Part model, mm, in its own coordinate system. Coordinates: 2 decimals unless noted, no trailing zeros. Loops run counter-clockwise (first coordinate to the right, second up) from the corner with the lowest first, then second, coordinate; pieces in that order, holes last. Notation, with made-up numbers: (-14, 51.25) -> (-4, 51.25) arc R22 cw to (-4, 65.25) -> close; hole circle Ø10 at (0.5, -38.5). An arc over 180 degrees is marked (long way). Use one line per item in the form item = value. Start each with the question number.
(1) Band-saw the part on D-D on z = 15.24. Give the cut face in (x, y) (3 decimals).
(2) Band-saw the part on C-C on x = 0. Give the cut face in (y, z) (3 decimals).
(3) Band-saw the part on A-A on z = 189. Give the cut face in (x, y) (3 decimals), then the cut area to 3 significant figures.
(4) Drill centre lines: L1, parallel to X at y = 4, z = 29.5 (3 decimals); L2, parallel to X at y = 11.6, z = 15.24. Where is each one in solid material? Low to high. Write a range as [from, to].
(5) Band-saw the part on B-B on y = 0. Give the cut face in (x, z) (3 decimals), then the cut area to 3 significant figures.
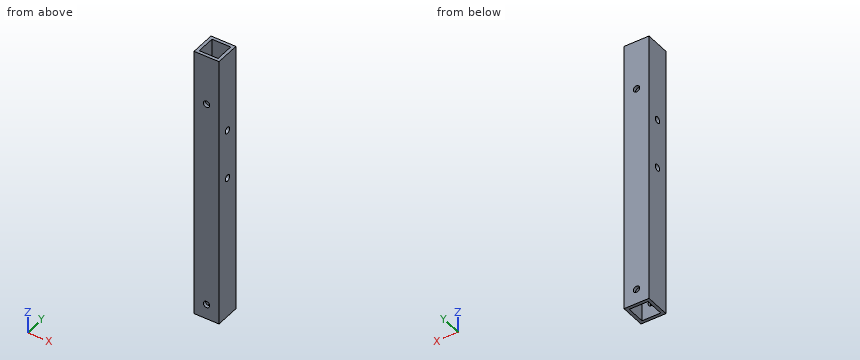
```python
from build123d import *

# Parameters (mm, degrees)
SKETCH2_W           = 25.4
SKETCH2_H           = 25.4
BOSS_EXTRUDE1_DEPTH = 279.4
SKETCH4_W           = 19.05
SKETCH4_H           = 19.05
CUT_EXTRUDE1_DEPTH  = 280.9766776
SKETCH5_R           = 3.2639
CUT_EXTRUDE2_DEPTH  = 281.839473721
SKETCH6_R           = 3.2639
CUT_EXTRUDE3_DEPTH  = 281.839473721
SKETCH8_R           = 3.2639
CUT_EXTRUDE5_DEPTH  = 281.839473721


with BuildPart() as part:
    # Sketch2 → Boss-Extrude1 (new body)
    with BuildSketch(Plane.XY):
        Rectangle(SKETCH2_W, SKETCH2_H)
    extrude(amount=BOSS_EXTRUDE1_DEPTH)

    # Sketch4 → Cut-Extrude1 (cut, through all)
    with BuildSketch(Plane.XY):
        Rectangle(SKETCH4_W, SKETCH4_H)
    extrude(amount=CUT_EXTRUDE1_DEPTH, mode=Mode.SUBTRACT)

    # Sketch5 → Cut-Extrude2 (cut, through all)
    with BuildSketch(Plane(origin=(0, 12.7, 0), x_dir=(1, 0, 0), z_dir=(0, 1, 0))):
        with Locations(Location((0, -15.24, 0), (0, 0, 270))):
            Circle(SKETCH5_R)
    extrude(amount=-CUT_EXTRUDE2_DEPTH, mode=Mode.SUBTRACT)

    # Sketch6 → Cut-Extrude3 (cut, through all)
    with BuildSketch(Plane(origin=(0, 12.7, 0), x_dir=(1, 0, 0), z_dir=(0, 1, 0))):
        with Locations(Location((0, -228.6, 0), (0, 0, 270))):
            Circle(SKETCH6_R)
    extrude(amount=-CUT_EXTRUDE3_DEPTH, mode=Mode.SUBTRACT)

    # Sketch8 → Cut-Extrude5 (cut, through all)
    with BuildSketch(Plane.ZY.offset(12.7)):
        with Locations((198.12, 0)):
            Circle(SKETCH8_R)
        with Locations((147.32, 0)):
            Circle(SKETCH8_R)
    extrude(amount=-CUT_EXTRUDE5_DEPTH, mode=Mode.SUBTRACT)


solid = part.part
```
A:
q1.outline = (-12.7, -12.7) -> (-3.264, -12.7) -> (-3.264, -9.525) -> (-9.525, -9.525) -> (-9.525, 9.525) -> (-3.264, 9.525) -> (-3.264, 12.7) -> (-12.7, 12.7) -> close; (3.264, -12.7) -> (12.7, -12.7) -> (12.7, 12.7) -> (3.264, 12.7) -> (3.264, 9.525) -> (9.525, 9.525) -> (9.525, -9.525) -> (3.264, -9.525) -> close
q2.outline = (-12.7, 0) -> (-9.525, 0) -> (-9.525, 11.976) -> (-12.7, 11.976) -> close; (-12.7, 18.504) -> (-9.525, 18.504) -> (-9.525, 225.336) -> (-12.7, 225.336) -> close; (-12.7, 231.864) -> (-9.525, 231.864) -> (-9.525, 279.4) -> (-12.7, 279.4) -> close; (9.525, 0) -> (12.7, 0) -> (12.7, 11.976) -> (9.525, 11.976) -> close; (9.525, 18.504) -> (12.7, 18.504) -> (12.7, 225.336) -> (9.525, 225.336) -> close; (9.525, 231.864) -> (12.7, 231.864) -> (12.7, 279.4) -> (9.525, 279.4) -> close
q3.outline = (-12.7, -12.7) -> (12.7, -12.7) -> (12.7, 12.7) -> (-12.7, 12.7) -> close; hole (-9.525, -9.525) -> (9.525, -9.525) -> (9.525, 9.525) -> (-9.525, 9.525) -> close
q3.area = 282 mm²
q4.L1 = [-12.7, -9.525], [9.525, 12.7]
q4.L2 = [-12.7, -3.26], [3.26, 12.7]
q5.outline = (-12.7, 0) -> (-9.525, 0) -> (-9.525, 144.056) -> (-12.7, 144.056) -> close; (-12.7, 150.584) -> (-9.525, 150.584) -> (-9.525, 194.856) -> (-12.7, 194.856) -> close; (-12.7, 201.384) -> (-9.525, 201.384) -> (-9.525, 279.4) -> (-12.7, 279.4) -> close; (9.525, 0) -> (12.7, 0) -> (12.7, 144.056) -> (9.525, 144.056) -> close; (9.525, 150.584) -> (12.7, 150.584) -> (12.7, 194.856) -> (9.525, 194.856) -> close; (9.525, 201.384) -> (12.7, 201.384) -> (12.7, 279.4) -> (9.525, 279.4) -> close
q5.area = 1,690 mm²
